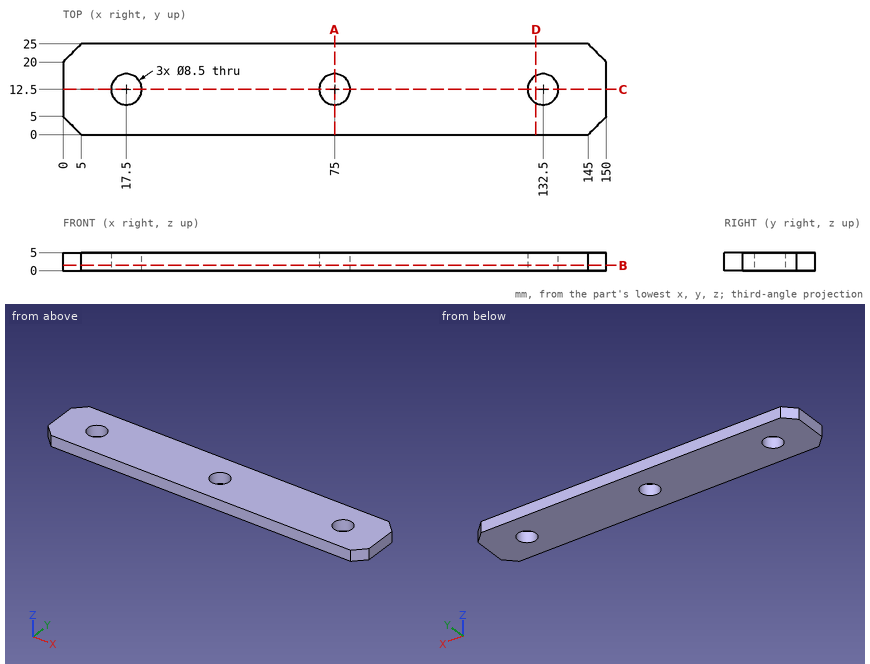
The drawing under review shows one solid part. Ordinate dimensions are in mm from its lowest x, y, z. Give positions to 0.01 mm unless a question says otherwise; leave off trailing zeros. Order: outer loops, then holes, each group sorted by start corner. A loop starts at its lowest first (then second) coordinate and runs counter-clockwise, first axis right, second up. Notation, with made-up numbers: M 6.25,36 L 12.25,36 A16 cw 12.25,62 Z; hole C 80,47.5 d10. An arc over 180 degrees is marked long. Answer in a Markdown table with one row per item. Add a question column.
1. Add section B-B on z = 1.45. State the section outline as (x, y) points.
2. Add section C-C on y = 12.5. State the section outline as (x, z) points.
3. Add section D-D on x = 130.5. State the section outline as (y, z) points, plus the area to 3 significant figures.
4. To check wall thickness, follow line 1 along Y through (x, z) = (17.5, 3.05); line 2 along Y through (x, z) = (134.5, 2.6); line 3 along X through (y, z) = (10.25, 2.3). State the ranges of each line that lie inside material, in increasing order.
5. For pin 1 Ø7 at (x, y) = (132.5, 12.5) entering from +Z, flat-tipped, find the tip position at first contact; note if it passes through.
6. Add section A-A on x = 75. State the section outline as (y, z) points.
The answers:
| question | item | result |
|---|---|---|
| 1 | outline | M 0,5 L 5,0 L 145,0 L 150,5 L 150,20 L 145,25 L 5,25 L 0,20 Z; hole C 17.5,12.5 d8.5; hole C 75,12.5 d8.5; hole C 132.5,12.5 d8.5 |
| 2 | outline | M 0,0 L 13.25,0 L 13.25,5 L 0,5 Z; M 21.75,0 L 70.75,0 L 70.75,5 L 21.75,5 Z; M 79.25,0 L 128.25,0 L 128.25,5 L 79.25,5 Z; M 136.75,0 L 150,0 L 150,5 L 136.75,5 Z |
| 3 | outline | M 0,0 L 8.75,0 L 8.75,5 L 0,5 Z; M 16.25,0 L 25,0 L 25,5 L 16.25,5 Z |
| 3 | area | 87.5 mm2 |
| 4 | line 1 | 0 to 8.25, 16.75 to 25 |
| 4 | line 2 | 0 to 8.75, 16.25 to 25 |
| 4 | line 3 | 0 to 13.89, 21.11 to 71.39, 78.61 to 128.89, 136.11 to 150 |
| 5 | pin 1 | through |
| 6 | outline | M 0,0 L 8.25,0 L 8.25,5 L 0,5 Z; M 16.75,0 L 25,0 L 25,5 L 16.75,5 Z |
